Could you check a few things on this model? Use its own coordinates, in mm. A direction names the side the tool comes from. Round coordinates to 2 decimals unless told otherwise and drop trailing zeros. One line per item, written item: value.
from build123d import *

# Parameters (mm, degrees)
SKETCH1_R           = 20.6375
SKETCH1_R_2         = 17.4625
BOSS_EXTRUDE1_DEPTH = 3.175
THREAD1_PITCH       = 1.058333333
CUT_EXTRUDE1_DEPTH  = 30.47257683
CIRPATTERN1_COUNT   = 4


with BuildPart() as part:
    # Sketch1 → Boss-Extrude1 (new body)
    with BuildSketch(Plane(origin=(0, 0, 0), x_dir=(0, 0, -1), z_dir=(1, 0, 0))):
        Circle(SKETCH1_R)
        Circle(SKETCH1_R_2, mode=Mode.SUBTRACT)
    extrude(amount=BOSS_EXTRUDE1_DEPTH)

    # Thread1: the profile of Thread Profile1 profile screwed along a right-hand helix of 3 turns, 8 arcs to a turn; built about Z, then put on its axis
    thread1_z = Axis((0, 0, 0), (0, 0, 1))
    thread1_corners = [(17.4628, 0, -0.000173205), (17.4628, 0, 0.926214869), (16.889660282, 0, 0.595312499), (16.889660282, 0, 0.330729165)]
    with BuildLine(mode=Mode.PRIVATE) as thread1_profile:
        Line(thread1_corners[0], thread1_corners[1])
        Line(thread1_corners[1], thread1_corners[2])
        Line(thread1_corners[2], thread1_corners[3])
        Line(thread1_corners[3], thread1_corners[0])
    thread1_cap = Face(thread1_profile.wire())
    thread1_turn_angles = [0, 22.5, 45, 67.5, 90, 112.5, 135, 157.5, 180, 202.5, 225, 247.5, 270, 292.5, 315, 337.5, 360]
    thread1_turn_weights = [1, 0.9238795325112867, 1, 0.9238795325112867, 1, 0.9238795325112867, 1, 0.9238795325112867, 1, 0.9238795325112867, 1, 0.9238795325112867, 1, 0.9238795325112867, 1, 0.9238795325112867, 1]
    thread1_turn_rails = [Edge.make_bspline([Vector(p[0], p[1], 0).rotate(thread1_z, thread1_turn_angles[k]) / thread1_turn_weights[k] + Vector(0, 0, p[2] + THREAD1_PITCH * thread1_turn_angles[k] / 360) for k in range(17)], [0, 0, 0, 1, 1, 2, 2, 3, 3, 4, 4, 5, 5, 6, 6, 7, 7, 8, 8, 8], 2, thread1_turn_weights) for p in thread1_corners]
    thread1_turn_sides = [Face.make_surface_from_curves(thread1_turn_rails[p[0]], thread1_turn_rails[p[1]]) for p in [(0, 1), (1, 2), (2, 3), (3, 0)]]
    thread1 = Plane(origin=(3.175, 0, 0), x_dir=(0, 0, 1), z_dir=(-1, 0, 0)) * Solid(Shell([*[p.moved(Location((0, 0, THREAD1_PITCH * i))) for i in range(3) for p in thread1_turn_sides], thread1_cap, thread1_cap.rotate(thread1_z, 1080).moved(Location((0, 0, THREAD1_PITCH * 1080 / 360)))]))
    add(thread1)

    # Sketch4 → Cut-Extrude1 (cut, symmetric)
    with BuildSketch(Plane(origin=(3.175, 0, 0), x_dir=(0, 0, -1), z_dir=(1, 0, 0))):
        Polygon((-1.5875, 124.225317778), (-1.5875, 20.576351717), (-1.5875, 19.05), (1.5875, 19.05), (1.5875, 20.576351717), (1.5875, 124.225317778), (1.5875, 331.523249901), (-1.5875, 331.523249901), align=None)
    cut_extrude1 = extrude(amount=CUT_EXTRUDE1_DEPTH, both=True, mode=Mode.SUBTRACT)

    # CirPattern1: Cut-Extrude1 ×4 about axis
    cirpattern1_axis = Axis((-17.546691261, 0, 0), (1, 0, 0))
    for i in range(1, CIRPATTERN1_COUNT):
        add(cut_extrude1.rotate(cirpattern1_axis, i * 360 / CIRPATTERN1_COUNT), mode=Mode.SUBTRACT)


solid = part.part
(1) I'm going to push flat-ended pins straight in: pin 1 Ø1.6 at (x, z) = (1.5, 0) entering from -Y; pin 2 Ø1.7 at (x, y) = (1, 20) entering from +Z; pin 3 Ø1.2 at (x, z) = (2, 19.5) entering from -Y; pin 4 Ø10 at (y, z) = (-3.5, 8) entering from +X. Where does each tip first touch, or does it pass through?
Recorded:
pin 1: y = -19.05
pin 2: z = 7.69
pin 3: y = -8.29
pin 4: through
(2) If I drill on L1, parallel to Y at x = 1.4, z = 0; L2, parallel to Y at x = 0.1, z = -7.5; L3, parallel to Z at x = 0.3, y = -11, over which ranges is the centre line in solid material (lowest first)?
Recorded:
L1: -19.05 to -17.46, 16.89 to 19.05
L2: -19.23 to -15.31, 15.17 to 19.23
L3: -17.46 to -13.31, 13.45 to 17.46
(3) For faces 1 (the face through (2, 19.05, 0)), 2 (the face through (1.565, 14.447, -14.737)), 3 (the face through (2, -20, 1.588)), 4 (the face through (2, 0, -19.05)), 5 (the face through (2, 1.588, 20)), which set-ups out of +Z, -Z, +X, -X, +Y, -Y let a thin tool reach every point of the face, with its end or its side?
Recorded:
face 1: +X, -X, +Y
face 2: -Z, +X, -X, +Y
face 3: +X, -X, -Y
face 4: -Z, +X, -X
face 5: +Z, +X, -X
(4) Thinking about a two-plate mould opening in Y: for faces 6 (the face through (0, 5, 17)), 7 (the face through (1.565, -14.447, 14.737)), 8 (the face through (2, 0, 19.05)), which applies, released by +Y, released by -Y, zero draft, split by the parting line, or undercut?
Recorded:
face 6: zero draft
face 7: released by -Y
face 8: undercut
